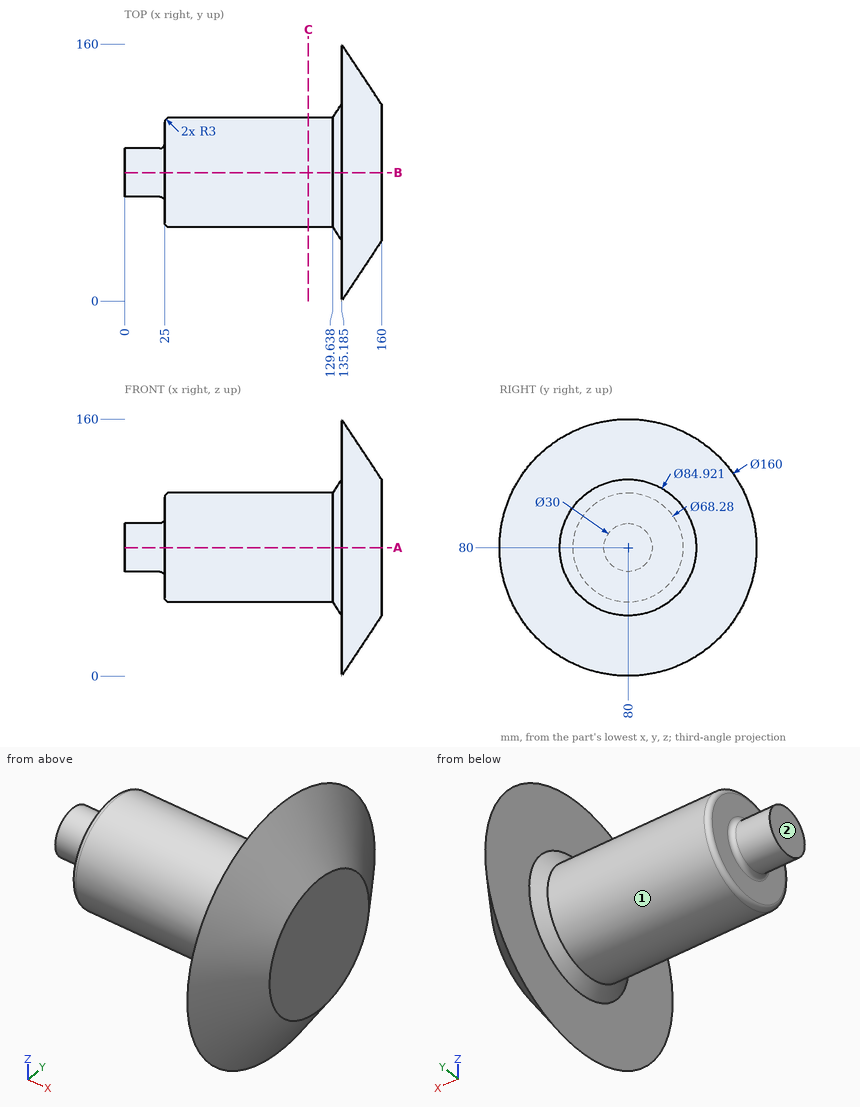
Input: dimensioned drawing with shaded views. Units: mm. Origin: part minimum x, y, z. A direction names the side the tool comes from. Round coordinates to 2 decimals unless told otherwise and drop trailing zeros. Order: outer loops, then holes, each group sorted by start corner. A loop starts at its lowest first (then second) coordinate and runs counter-clockwise, first axis right, second up.
Q1. Material intervals for probe 1 along Y at (x, z) = (21.5, 81); probe 2 along Y at (x, z) = (47, 80.5); probe 3 along X at (y, z) = (29.5, 96.5) (1 decimal), sorted ascending.
Result sheet:
probe 1: y = 65.03 to 94.97
probe 2: y = 45.86 to 114.14
probe 3: x = 135.2 to 152.9
Q2. Section C-C, the plane x = 114.5. Output: boundary loops of the cut face in (y, z).
Result sheet:
outline: circle Ø68.28 at (80, 80)
Q3. Access query for the marked faces 1 and 2. Directions: +Z, -Z, +X, -X, +Y, -Y. A direction counts if a zero-diameter tool reaches every point of the face in a straight line with its end or side. Return the directions, or none.
Result sheet:
face 1: -X
face 2: +Z, -Z, -X, +Y, -Y
Q4. Pin query (flat end, axial travel): pin 1 (10 mm diameter, centred on y = 126.5, z = 34, fed in from -X) (3 decimals); pin 2 (4 mm diameter, centred on x = 78, z = 72.5, fed in from -Y); pin 3 (12 mm diameter, centred on y = 81, z = 28, fed in from +X). Return the tip coordinate at first contact, or that it passes through.
Result sheet:
pin 1: stops at x = 135.185
pin 2: stops at y = 46.31
pin 3: stops at x = 157.65
Q5. Section A-A, the plane z = 80. Output: boundary loops of the cut face in (x, y) (1 decimal).
Result sheet:
outline: (0, 65) - (22, 65) arc R3 cw to (25, 62) - (25, 48.9) arc R3 ccw to (28, 45.9) - (129.6, 45.9) - (135.2, 37.5) - (135.2, 0) - (160, 37.5) - (160, 122.5) - (135.2, 160) - (135.2, 122.5) - (129.6, 114.1) - (28, 114.1) arc R3 ccw to (25, 111.1) - (25, 98) arc R3 cw to (22, 95) - (0, 95) - close
